```python
from build123d import *

# Parameters (mm, degrees)
SKETCH1_W           = 30
SKETCH1_H           = 10
SKETCH1_R           = 1.5
BOSS_EXTRUDE1_DEPTH = 0.75
SKETCH2_R           = 1.5
SKETCH2_R_2         = 1
CUT_EXTRUDE1_DEPTH  = 1.5
BOSS_EXTRUDE3_START = -4.25
BOSS_EXTRUDE3_DEPTH = 0.75
SKETCH4_R           = 1
CUT_EXTRUDE2_DEPTH  = 10
FILLET1_R           = 1
BOSS_EXTRUDE4_START = 14
BOSS_EXTRUDE4_DEPTH = 1


with BuildPart() as part:
    # Sketch1 → Boss-Extrude1 (new body, symmetric)
    with BuildSketch(Plane(origin=(0, 0, 0), x_dir=(1, 0, 0), z_dir=(0, 1, 0))):
        Rectangle(SKETCH1_W, SKETCH1_H)
        with Locations((0, -2)):
            Circle(SKETCH1_R, mode=Mode.SUBTRACT)
    extrude(amount=BOSS_EXTRUDE1_DEPTH, both=True)

    # Sketch2 → Cut-Extrude1 (cut)
    with BuildSketch(Plane(origin=(0, 0.75, 0), x_dir=(1, 0, 0), z_dir=(0, 1, 0))):
        with Locations((-10, -2)):
            Circle(SKETCH2_R)
        with Locations((10, -2)):
            Circle(SKETCH2_R)
        with Locations((-5.5, -2)):
            Circle(SKETCH2_R_2)
        with Locations((5.5, -2)):
            Circle(SKETCH2_R_2)
    extrude(amount=-CUT_EXTRUDE1_DEPTH, mode=Mode.SUBTRACT)

    # Sketch3 → Boss-Extrude3 (add, symmetric)
    with BuildSketch(Plane.XY.offset(BOSS_EXTRUDE3_START)):
        Polygon((15, 0.75), (15, 20.75), (7, 20.75), (7, 6.75), (-7, 6.75), (-7, 20.75), (-15, 20.75), (-15, 0.75), align=None)
    extrude(amount=BOSS_EXTRUDE3_DEPTH, both=True)

    # Sketch4 → Cut-Extrude2 (cut)
    with BuildSketch(Plane.XY):
        with Locations((-11, 13.25)):
            Circle(SKETCH4_R)
        with Locations((11, 13.25)):
            Circle(SKETCH4_R)
    extrude(amount=-CUT_EXTRUDE2_DEPTH, mode=Mode.SUBTRACT)

    # Fillet1
    fillet1_edges = [part.edges().sort_by_distance(p)[0] for p in [
        (7, 6.75, -4.25),
        (-7, 6.75, -4.25),
    ]]
    fillet(fillet1_edges, radius=FILLET1_R)

    # Sketch7 → Boss-Extrude4 (add)
    with BuildSketch(Plane(origin=(0, 0, 0), x_dir=(0, 0, -1), z_dir=(1, 0, 0)).offset(BOSS_EXTRUDE4_START)):
        Polygon((3.5, 0.75), (3.5, 20.75), (0, 20.75), (-5, 9.840050856), (-5, 0.75), align=None)
    boss_extrude4 = extrude(amount=BOSS_EXTRUDE4_DEPTH)

    # Mirror1: Boss-Extrude4 across plane
    add(boss_extrude4.mirror(Plane(origin=(0, 0, 0), x_dir=(0, 0, 1), z_dir=(1, 0, 0))))


solid = part.part
```
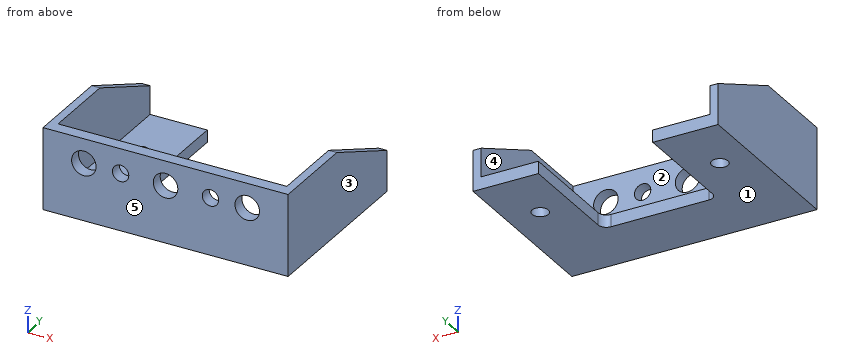
Can you work these out from the model? Positions are in its coordinate system, mm. Face numbers are marked on the shaded views. A direction names the side the tool comes from. Round coordinates to 2 decimals unless told otherwise and drop trailing zeros. Loops run counter-clockwise (first coordinate to the right, second up) from the corner with the lowest first, then second, coordinate; pieces in that order, holes last. Notation, with made-up numbers: (-16, 62.5) -> (18, 62.5) arc R30 cw to (18, 100.5) -> close; hole circle Ø7 at (-22, 52.5). An arc over 180 degrees is marked (long way). Answer in a Markdown table with one row per item.
Item 1: Will these pins go through, and if not, where does the flat tip stop? P1, Ø2.5, axis at x = -5.5, z = 2, coming from the +Y side; P2, Ø1.5, axis at x = -11.5, y = 18, coming from the +Z side.
Answer block:
| item | result |
|---|---|
| P1 | y = 0.75 |
| P2 | z = -3.5 |
Item 2: Suppose I cut it at C-C, the plane y = 11.25. List the corners of the cut face in (x, z) for me.
Answer block:
| item | result |
|---|---|
| outline | (-15, -5) -> (-7, -5) -> (-7, -3.5) -> (-14, -3.5) -> (-14, 4.35) -> (-15, 4.35) -> close; (7, -5) -> (15, -5) -> (15, 4.35) -> (14, 4.35) -> (14, -3.5) -> (7, -3.5) -> close |
Item 3: Suppose I cut it at B-B, the plane z = -4. List the corners of the cut face in (x, y) for me, plus the area to 3 significant figures.
Answer block:
| item | result |
|---|---|
| outline | (-15, -0.75) -> (15, -0.75) -> (15, 20.75) -> (7, 20.75) -> (7, 7.75) arc R1 cw to (6, 6.75) -> (-6, 6.75) arc R1 cw to (-7, 7.75) -> (-7, 20.75) -> (-15, 20.75) -> close; hole circle Ø2 at (-11, 13.25); hole circle Ø2 at (11, 13.25) |
| area | 443 mm² |
Item 4: Suppose I cut it at D-D, the plane z = 2. List the corners of the cut face in (x, y) for me, plus the area to 3 significant figures.
Answer block:
| item | result |
|---|---|
| outline | (-15, -0.75) -> (-11.5, -0.75) -> (-11.5, 0.75) -> (-14, 0.75) -> (-14, 16.39) -> (-15, 16.39) -> close; (-8.5, -0.75) -> (-6.5, -0.75) -> (-6.5, 0.75) -> (-8.5, 0.75) -> close; (-4.5, -0.75) -> (-1.5, -0.75) -> (-1.5, 0.75) -> (-4.5, 0.75) -> close; (1.5, -0.75) -> (4.5, -0.75) -> (4.5, 0.75) -> (1.5, 0.75) -> close; (6.5, -0.75) -> (8.5, -0.75) -> (8.5, 0.75) -> (6.5, 0.75) -> close; (11.5, -0.75) -> (15, -0.75) -> (15, 16.39) -> (14, 16.39) -> (14, 0.75) -> (11.5, 0.75) -> close |
| area | 56.8 mm² |
Item 5: We'd pull the mould along X, two halves only. Please class the marked faces 1, 2 and 3: released by +X, released by -X, zero draft, split by the parting line, or undercut.
Answer block:
| item | result |
|---|---|
| face 1 | zero draft |
| face 2 | undercut |
| face 3 | released by +X |
Item 6: Suppose I cut it at A-A, the plane x = 5.5. List the corners of the cut face in (y, z) for me, plus the area to 3 significant figures.
Answer block:
| item | result |
|---|---|
| outline | (-0.75, -5) -> (6.75, -5) -> (6.75, -3.5) -> (0.75, -3.5) -> (0.75, 1) -> (-0.75, 1) -> close; (-0.75, 3) -> (0.75, 3) -> (0.75, 5) -> (-0.75, 5) -> close |
| area | 21.0 mm² |
Item 7: On a 3-axis mill with a long thin cutter (end or side, diameter ignored), from which of +Z, -Z, +X, -X, +Y, -Y can I reach the whole of each face in a straight line? I mean the marked faces 4 and 5. Say none if no direction works.
Answer block:
| item | result |
|---|---|
| face 4 | +Z, +Y |
| face 5 | +Z, -Z, +X, -X, -Y |
Item 8: If I drill on probe 1 along X at (y, z) = (-0.1, 2); probe 2 along Z at (x, y) = (-10, 0.45); probe 3 along X at (y, z) = (10.25, -2.75), over which ranges is the centre line in solid material (lowest first)?
Answer block:
| item | result |
|---|---|
| probe 1 | -15 to -11.5, -8.5 to -6.5, -4.5 to -1.5, 1.5 to 4.5, 6.5 to 8.5, 11.5 to 15 |
| probe 2 | -5 to 0.5, 3.5 to 5 |
| probe 3 | -15 to -14, 14 to 15 |
